The figure shows three views and two pictorial views of one solid part (mm, origin at its lowest corner). Answer the questions. A direction names the side the tool comes from. Coordinates: 2 decimals unless noted, no trailing zeros. Write each loop counter-clockwise with the first axis right and the second up, starting at its lowest first coordinate (ties: lowest second). Pieces come first, ordered by that corner, then holes. Notation, with made-up numbers: M 62,13 L 102,13 A21 ccw 102,32 Z; hole C 35.25,61.25 d11. An arc over 180 degrees is marked long. Write item = value, one per line. Start each with the question number.
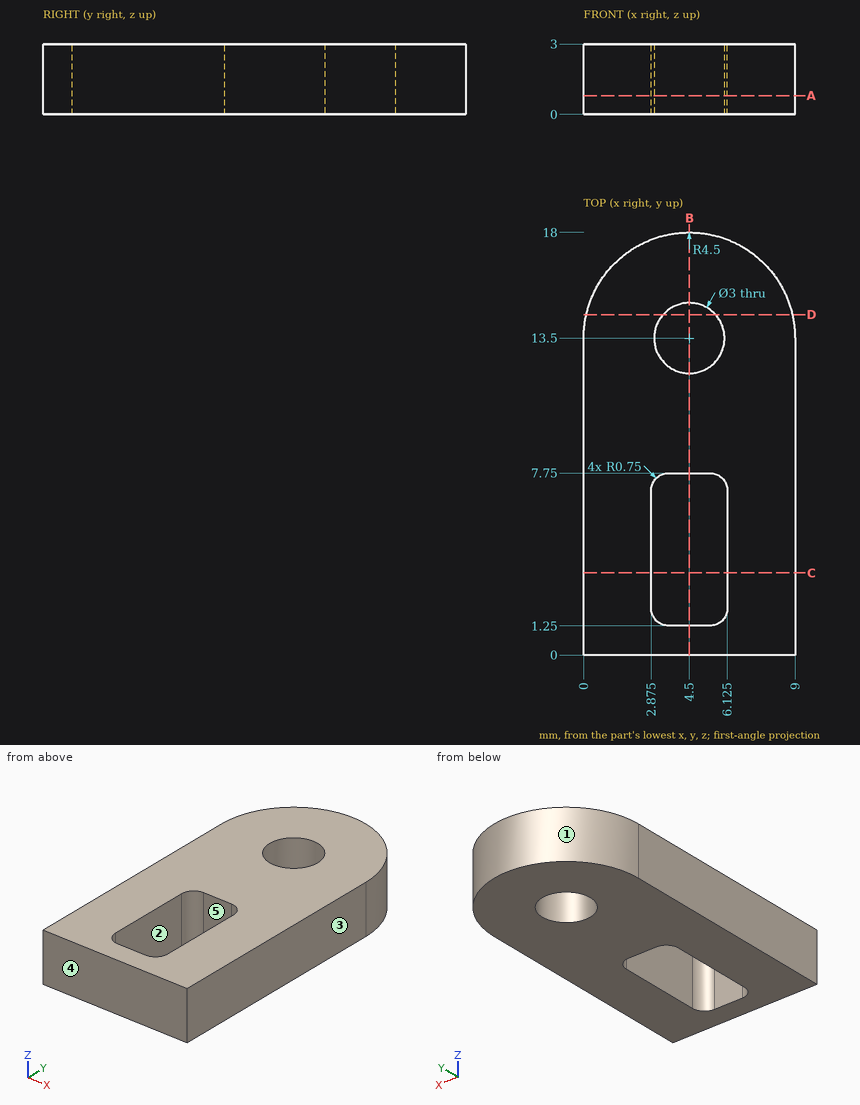
1. The part is cut by section C-C, the plane y = 3.5. Write down the section's boundary in (x, z) (3 decimals), and give its area (4 significant figures).
2. This flat-tipped pin is pushed along its axis until it touches: pin 1 (2.5 mm diameter, centred on x = 4.5, y = 13.5, fed in from +Z). Where does it stop, or does it pass through?
3. For a pull along Y with two mould halves and no side action, classify the marked faces 3, 4 and 5 as pulls with the +Y half, pulls with the -Y half, needs draft (parallel to the pull), parting line crosses it, or undercut.
4. The part is cut by section B-B, the plane x = 4.5. Write down the section's boundary in (y, z).
5. Straight lines are drawn through the part: L1, parallel to Y at x = 4.5, z = 1.55; L2, parallel to X at y = 4, z = 0.45 (3 decimals); L3, parallel to Y at x = 4, z = 0.7. For each, find the intervals that lie inside material, in ascending order. Write a range as [from, to].
6. The part is cut by section A-A, the plane z = 0.8. Write down the section's boundary in (x, y) (3 decimals).
7. The part is cut by section D-D, the plane y = 14.5. Write down the section's boundary in (x, z).
8. For the marked faces 1 and 2, determine the directions among +Z, -Z, +X, -X, +Y, -Y from which every point of the face is accessible in a straight line to the end or side of a thin tool.
Solution:
q1.outline = M 0,0 L 2.875,0 L 2.875,3 L 0,3 Z; M 6.125,0 L 9,0 L 9,3 L 6.125,3 Z
q1.area = 17.25 mm^2
q2.pin_1 = through
q3.face_3 = needs draft
q3.face_4 = pulls with the -Y half
q3.face_5 = undercut
q4.outline = M 0,0 L 1.25,0 L 1.25,3 L 0,3 Z; M 7.75,0 L 12,0 L 12,3 L 7.75,3 Z; M 15,0 L 18,0 L 18,3 L 15,3 Z
q5.L1 = [0, 1.25], [7.75, 12], [15, 18]
q5.L2 = [0, 2.875], [6.125, 9]
q5.L3 = [0, 1.25], [7.75, 12.09], [14.91, 17.97]
q6.outline = M 0,0 L 9,0 L 9,13.5 A4.5 ccw 0,13.5 Z; hole M 2.875,2 A0.75 ccw 3.625,1.25 L 5.375,1.25 A0.75 ccw 6.125,2 L 6.125,7 A0.75 ccw 5.375,7.75 L 3.625,7.75 A0.75 ccw 2.875,7 Z; hole C 4.5,13.5 d3
q7.outline = M 0.11,0 L 3.38,0 L 3.38,3 L 0.11,3 Z; M 5.62,0 L 8.89,0 L 8.89,3 L 5.62,3 Z
q8.face_1 = +Z, -Z, +Y
q8.face_2 = +Z, -Z
